Check sheet for the modelled part. Datum: model origin and axes. Units: mm. Face numbers are marked on the shaded views. A direction names the side the tool comes from. Coordinates: 2 decimals unless noted, no trailing zeros. Loops run counter-clockwise (first coordinate to the right, second up) from the corner with the lowest first, then second, coordinate; pieces in that order, holes last. Notation, with made-up numbers: (-10, -18.75) - (35, -18.75) arc R25 cw to (35, 8.25) - close; hole circle Ø6 at (-34, -9). An arc over 180 degrees is marked (long way). Use a Markdown table: item, result. Add a question column.
1) Tool access check on the marked faces 1, 2, 3 and 4. Record the directions out of +Z, -Z, +X, -X, +Y, -Y that give a thin tool (end or side, any length) a straight path to the whole face; none if there is none.
2) Sectioned sample at A-A, the plane z = 10. Enter the section's corners in (x, y), then the cut area to 3 significant figures.
3) Go/stop test with flat-tipped pins: P1, Ø6, axis at y = -25.5, z = -2, coming from the -X side; P2, Ø6, axis at x = 3.5, y = 35, coming from the -Z side; P3, Ø7.5, axis at y = 47, z = 11, coming from the +X side. Record where each tip stops, or that it passes through.
4) Sectioned sample at D-D, the plane z = 23.5. Enter the section's corners in (x, y).
5) Sectioned sample at C-C, the plane y = 10.5. Enter the section's corners in (x, z), then the cut area to 3 significant figures.
6) Draft check along Y on the marked faces 5, 6 and 7. Enter one of: pulls with the +Y half, pulls with the -Y half, needs draft (parallel to the pull), parting line crosses it, or undercut.
7) Sectioned sample at B-B, the plane x = 0. Enter the section's corners in (y, z), then the cut area to 3 significant figures.
8) Thickness scan on line 1 (Y direction, x = -16.5, z = 10); line 2 (X direction, y = -2.5, z = 8); line 3 (X direction, y = 59, z = 14.5). Record the ranges inside material, lowest first.
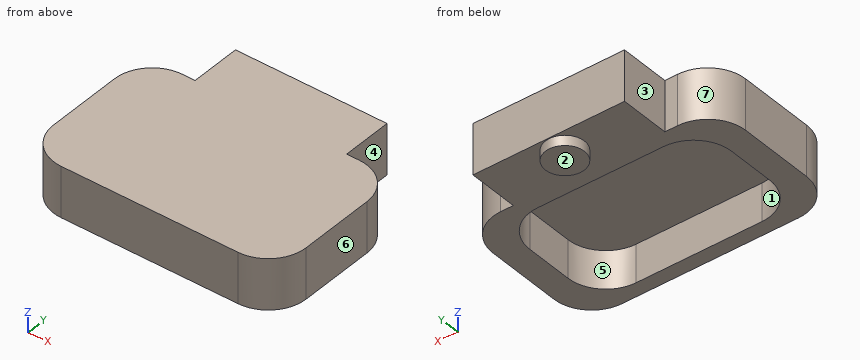
from build123d import *

# Parameters (mm, degrees)
F0_W     = 76.2
F0_H     = 25.326092267
F1_DEPTH = 25.4
F2_DEPTH = 19.05
F3_R     = 9.771245389
F4_DEPTH = 5.08


with BuildPart() as f1:
    # F0 (on Top) → F1 (new body)
    with BuildSketch(Plane.XY):
        with BuildLine():
            ThreePointArc((-63.5, -19.05), (-57.9203841816, -32.5203841816), (-44.45, -38.1))
            Line((-44.45, -38.1), (44.45, -38.1))
            ThreePointArc((44.45, -38.1), (57.9203841816, -32.5203841816), (63.5, -19.05))
            Line((63.5, -19.05), (63.5, 19.05))
            ThreePointArc((63.5, 19.05), (57.9203841816, 32.5203841816), (44.45, 38.1))
            Line((44.45, 38.1), (38.1, 38.1))
            Line((38.1, 38.1), (-38.1, 38.1))
            Line((-38.1, 38.1), (-44.45, 38.1))
            ThreePointArc((-44.45, 38.1), (-57.9203841816, 32.5203841816), (-63.5, 19.05))
            Line((-63.5, 19.05), (-63.5, -19.05))
        make_face()
        with BuildLine():
            ThreePointArc((-50.7219098508, 11.9470546514), (-45.1422940324, 25.417438833), (-31.6719098508, 30.9970546514))
            Line((-31.6719098508, 30.9970546514), (31.6719098508, 30.9970546514))
            ThreePointArc((31.6719098508, 30.9970546514), (45.1422940324, 25.417438833), (50.7219098508, 11.9470546514))
            Line((50.7219098508, 11.9470546514), (50.7219098508, -11.9470546514))
            ThreePointArc((50.7219098508, -11.9470546514), (45.1422940324, -25.417438833), (31.6719098508, -30.9970546514))
            Line((31.6719098508, -30.9970546514), (-31.6719098508, -30.9970546514))
            ThreePointArc((-31.6719098508, -30.9970546514), (-45.1422940324, -25.417438833), (-50.7219098508, -11.9470546514))
            Line((-50.7219098508, -11.9470546514), (-50.7219098508, 11.9470546514))
        make_face(mode=Mode.SUBTRACT)
        with BuildLine():
            Line((31.6719098508, 30.9970546514), (-31.6719098508, 30.9970546514))
            ThreePointArc((-31.6719098508, 30.9970546514), (-45.1422940324, 25.417438833), (-50.7219098508, 11.9470546514))
            Line((-50.7219098508, 11.9470546514), (-50.7219098508, -11.9470546514))
            ThreePointArc((-50.7219098508, -11.9470546514), (-45.1422940324, -25.417438833), (-31.6719098508, -30.9970546514))
            Line((-31.6719098508, -30.9970546514), (31.6719098508, -30.9970546514))
            ThreePointArc((31.6719098508, -30.9970546514), (45.1422940324, -25.417438833), (50.7219098508, -11.9470546514))
            Line((50.7219098508, -11.9470546514), (50.7219098508, 11.9470546514))
            ThreePointArc((50.7219098508, 11.9470546514), (45.1422940324, 25.417438833), (31.6719098508, 30.9970546514))
        make_face()
        with Locations((0, 50.7630461335)):
            Rectangle(F0_W, F0_H)
    extrude(amount=F1_DEPTH)

    # F0 (on Top) → F2 (cut)
    with BuildSketch(Plane.XY):
        with BuildLine():
            Line((31.6719098508, 30.9970546514), (-31.6719098508, 30.9970546514))
            ThreePointArc((-31.6719098508, 30.9970546514), (-45.1422940324, 25.417438833), (-50.7219098508, 11.9470546514))
            Line((-50.7219098508, 11.9470546514), (-50.7219098508, -11.9470546514))
            ThreePointArc((-50.7219098508, -11.9470546514), (-45.1422940324, -25.417438833), (-31.6719098508, -30.9970546514))
            Line((-31.6719098508, -30.9970546514), (31.6719098508, -30.9970546514))
            ThreePointArc((31.6719098508, -30.9970546514), (45.1422940324, -25.417438833), (50.7219098508, -11.9470546514))
            Line((50.7219098508, -11.9470546514), (50.7219098508, 11.9470546514))
            ThreePointArc((50.7219098508, 11.9470546514), (45.1422940324, 25.417438833), (31.6719098508, 30.9970546514))
        make_face()
    extrude(amount=F2_DEPTH, mode=Mode.SUBTRACT)

    # F3 (on face) → F4 (join)
    with BuildSketch(Plane(origin=(0, 0, 0), x_dir=(1, 0, 0), z_dir=(0, 0, -1))):
        with Locations((0, -53.2785505056)):
            Circle(F3_R)
    extrude(amount=F4_DEPTH)


solid = f1.part
Solved:
| question | item | result |
|---|---|---|
| 1 | face 1 | -Z |
| 1 | face 2 | -Z, +X, -X, +Y, -Y |
| 1 | face 3 | +Z, -Z, -X, +Y |
| 1 | face 4 | +Z, -Z, +X, +Y |
| 2 | outline | (-63.5, -19.05) arc R19.05 ccw to (-44.45, -38.1) - (44.45, -38.1) arc R19.05 ccw to (63.5, -19.05) - (63.5, 19.05) arc R19.05 ccw to (44.45, 38.1) - (38.1, 38.1) - (38.1, 63.43) - (-38.1, 63.43) - (-38.1, 38.1) - (-44.45, 38.1) arc R19.05 ccw to (-63.5, 19.05) - close; hole (-50.72, -11.95) arc R19.05 ccw to (-31.67, -31) - (31.67, -31) arc R19.05 ccw to (50.72, -11.95) - (50.72, 11.95) arc R19.05 ccw to (31.67, 31) - (-31.67, 31) arc R19.05 ccw to (-50.72, 11.95) - close |
| 2 | area | 5,320 mm2 |
| 3 | P1 | stops at x = -63.03 |
| 3 | P2 | stops at z = 0 |
| 3 | P3 | stops at x = 38.1 |
| 4 | outline | (-63.5, -19.05) arc R19.05 ccw to (-44.45, -38.1) - (44.45, -38.1) arc R19.05 ccw to (63.5, -19.05) - (63.5, 19.05) arc R19.05 ccw to (44.45, 38.1) - (38.1, 38.1) - (38.1, 63.43) - (-38.1, 63.43) - (-38.1, 38.1) - (-44.45, 38.1) arc R19.05 ccw to (-63.5, 19.05) - close |
| 5 | outline | (-63.5, 0) - (-50.72, 0) - (-50.72, 19.05) - (50.72, 19.05) - (50.72, 0) - (63.5, 0) - (63.5, 25.4) - (-63.5, 25.4) - close |
| 5 | area | 1,290 mm2 |
| 6 | face 5 | undercut |
| 6 | face 6 | needs draft |
| 6 | face 7 | pulls with the +Y half |
| 7 | outline | (-38.1, 0) - (-31, 0) - (-31, 19.05) - (31, 19.05) - (31, 0) - (43.51, 0) - (43.51, -5.08) - (63.05, -5.08) - (63.05, 0) - (63.43, 0) - (63.43, 25.4) - (-38.1, 25.4) - close |
| 7 | area | 1,500 mm2 |
| 8 | line 1 | y = -38.1 to -31, 31 to 63.43 |
| 8 | line 2 | x = -63.5 to -50.72, 50.72 to 63.5 |
| 8 | line 3 | x = -38.1 to 38.1 |
